from build123d import *

# Parameters (mm, degrees)
SKIZZE1_W                       = 35
SKIZZE1_H                       = 85
AUFSATZ_LINEAR_AUSTRAGEN1_DEPTH = 40
SKIZZE2_R                       = 12.384443891
AUFSATZ_LINEAR_AUSTRAGEN2_DEPTH = 10
SKIZZE3_W                       = 20
SKIZZE3_H                       = 200
AUFSATZ_LINEAR_AUSTRAGEN3_DEPTH = 20


with BuildPart() as part:
    # Skizze1 → Aufsatz-Linear austragen1 (new body)
    with BuildSketch(Plane.XY):
        Rectangle(SKIZZE1_W, SKIZZE1_H)
    extrude(amount=-AUFSATZ_LINEAR_AUSTRAGEN1_DEPTH)

    # Skizze2 → Aufsatz-Linear austragen2 (add)
    with BuildSketch(Plane(origin=(0, 42.5, 0), x_dir=(1, 0, 0), z_dir=(0, 1, 0))):
        with Locations((0, 14.316526297)):
            Circle(SKIZZE2_R)
    extrude(amount=AUFSATZ_LINEAR_AUSTRAGEN2_DEPTH)

    # Skizze3 → Aufsatz-Linear austragen3 (add)
    with BuildSketch(Plane(origin=(0, 0, -40), x_dir=(-1, 0, 0), z_dir=(0, 0, -1))):
        with Locations((0, 57.5)):
            Rectangle(SKIZZE3_W, SKIZZE3_H)
    extrude(amount=AUFSATZ_LINEAR_AUSTRAGEN3_DEPTH)


solid = part.part
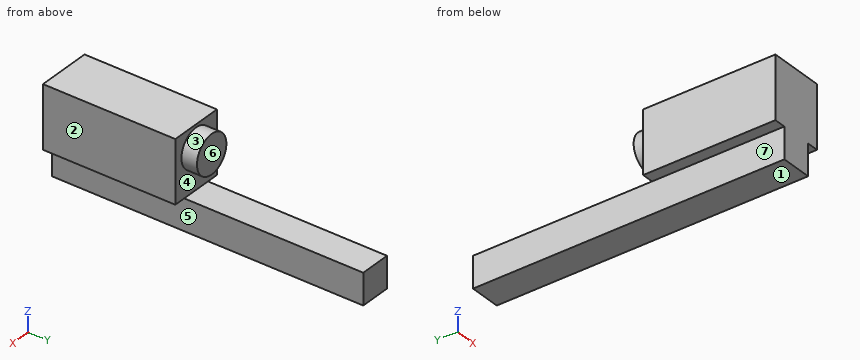
Design review of the part built by this model. Coordinates are the model's own, in mm. Face numbers are marked on the shaded views. A direction names the side the tool comes from. Coordinates: 2 decimals unless noted, no trailing zeros. Order: outer loops, then holes, each group sorted by start corner. A loop starts at its lowest first (then second) coordinate and runs counter-clockwise, first axis right, second up.
Item 1: Take a section at B-B, the plane x = 0. Write out the cut boundary in (y, z), then the cut area to 3 significant figures.
Item 2: For line 1 (Y direction, x = 7, z = -5.5); line 2 (X direction, y = 112, z = -49); line 3 (Y direction, x = -3, z = -33.5), list the stretches that pass through material, from the lowest coordinate up.
Item 3: Take a section at A-A, the plane y = 0.5. Write out the cut boundary in (x, z), then the cut area to 3 significant figures.
Item 4: Take a section at D-D, the plane z = -55.5. Write out the cut boundary in (x, y), then the cut area to 3 significant figures.
Item 5: Take a section at C-C, the plane z = -16.5. Write out the cut boundary in (x, y), then the cut area to 3 significant figures.
Item 6: For pin 1 Ø12 at (x, z) = (6.5, -19) entering from +Y; pin 2 Ø2 at (x, y) = (-15.5, 7.5) entering from -Z; pin 3 Ø10 at (y, z) = (63, -48.5) entering from +X, all flat-tipped, find the tip position at first contact; note any pin that passes through.
Item 7: For the marked faces 4, 5, 6 and 7, list the 3-axis set-ups (+Z, -Z, +X, -X, +Y, -Y) from which the entire face can be reached by the end or side of a thin tool; tool diameter is ignored.
Item 8: The part is to be moulded in two halves that separate along Z. For the marked faces 1, 2 and 3, say which applies: pulls with the +Z half, pulls with the -Z half, needs draft (parallel to the pull), parting line crosses it, or undercut.
The answers:
1. outline: (-42.5, -60) - (157.5, -60) - (157.5, -40) - (42.5, -40) - (42.5, -26.7) - (52.5, -26.7) - (52.5, -1.93) - (42.5, -1.93) - (42.5, 0) - (-42.5, 0) - close
1. area: 7,650 mm2
2. line 1: y = -42.5 to 52.5
2. line 2: x = -10 to 10
2. line 3: y = -42.5 to 42.5
3. outline: (-17.5, -40) - (-10, -40) - (-10, -60) - (10, -60) - (10, -40) - (17.5, -40) - (17.5, 0) - (-17.5, 0) - close
3. area: 1,800 mm2
4. outline: (-10, -42.5) - (10, -42.5) - (10, 157.5) - (-10, 157.5) - close
4. area: 4,000 mm2
5. outline: (-17.5, -42.5) - (17.5, -42.5) - (17.5, 42.5) - (12.19, 42.5) - (12.19, 52.5) - (-12.19, 52.5) - (-12.19, 42.5) - (-17.5, 42.5) - close
5. area: 3,220 mm2
6. pin 1: stops at y = 52.5
6. pin 2: stops at z = -40
6. pin 3: stops at x = 10
7. face 4: +Y
7. face 5: -Z, +X, +Y, -Y
7. face 6: +Z, +X, -X, +Y
7. face 7: -Z, -X, +Y, -Y
8. face 1: pulls with the -Z half
8. face 2: needs draft
8. face 3: undercut
